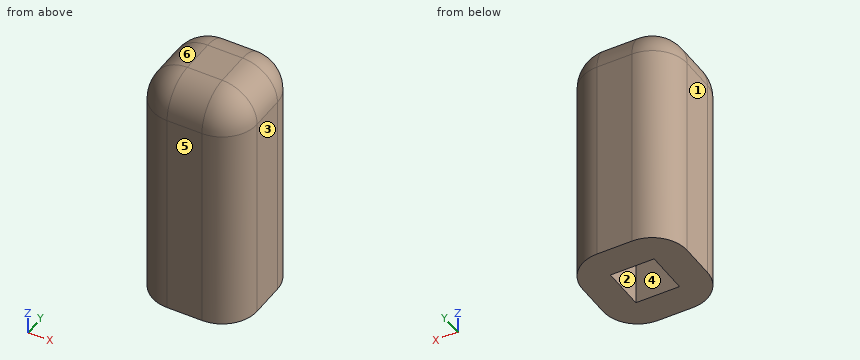
Autodesk Inventor part; units mm, degrees
ref_plane "YZ Plane" through (0, 0, 0) normal (1, 0, 0) x (0, 1, 0)
ref_plane "XZ Plane" through (0, 0, 0) normal (0, 1, 0) x (-1, 0, 0)
ref_plane "XY Plane" through (0, 0, 0) normal (0, 0, 1) x (1, 0, 0)
sketch "Sketch1" plane through (0, 0, 0) normal (0, 0, 1) x (1, 0, 0)
  line L0 (-1, 1) -> (1, 1)
  line L1 (1, 1) -> (1, -1)
  line L2 (1, -1) -> (-1, -1)
  line L3 (-1, -1) -> (-1, 1)
  line L4 (-1, 1) -> (1, -1) construction
  line L5 (1, 1) -> (-1, -1) construction
  line L6 (3, 3) -> (-3, 3)
  line L7 (-3, 3) -> (-3, -3)
  line L8 (-3, -3) -> (3, -3)
  line L9 (3, -3) -> (3, 3)
  point P0 (0, 0)
  dimension "d0" = 2
  dimension "d1" = 2
  dimension "d2" = 2
extrude "Extrusion1" add sketch "Sketch1" along normal blind 14
sketch "Sketch2" plane through (0, 0, 14) normal (0, 0, 1) x (1, 0, 0)
  line L0 (-3, -3) -> (3, -3)
  line L1 (3, -3) -> (3, 3)
  line L2 (3, 3) -> (-3, 3)
  line L3 (-3, 3) -> (-3, -3)
  line L4 (1, -1) -> (-1, -1)
  line L5 (-1, -1) -> (-1, 1)
  line L6 (-1, 1) -> (1, 1)
  line L7 (1, 1) -> (1, -1)
  point P0 (0, 0)
extrude "Extrusion2" add sketch "Sketch2" against normal blind 8 contours L4 L5 L6 L7
fillet "Fillet1" radius 2 8 edges at (3, 3, 7) (-3, 3, 7) (-3, -3, 7) (3, -3, 7) (3, 0, 14) (0, -3, 14) (-3, 0, 14) (0, 3, 14)
sketch "Sketch3" plane through (0, 0, 0) normal (0, 0, -1) x (-1, 0, 0)
  arc A0 (1, -3) -> (3, -1) centre (1, -1) ccw
  line L0 (3, 1) -> (3, -1)
  arc A1 (3, 1) -> (1, 3) centre (1, 1) ccw
  line L1 (-1, 3) -> (1, 3)
  arc A2 (-1, 3) -> (-3, 1) centre (-1, 1) ccw
  line L2 (-3, -1) -> (-3, 1)
  arc A3 (-3, -1) -> (-1, -3) centre (-1, -1) ccw
  line L3 (1, -3) -> (-1, -3)
  line L4 (-1, -1) -> (1, -1)
  line L5 (-1, 1) -> (-1, -1)
  line L6 (1, 1) -> (-1, 1)
  line L7 (1, -1) -> (1, 1)
  line L8 (-1.25, -1.25) -> (1.25, -1.25)
  line L9 (1.25, -1.25) -> (1.25, 1.25)
  line L10 (1.25, 1.25) -> (-1.25, 1.25)
  line L11 (-1.25, 1.25) -> (-1.25, -1.25)
  point P0 (0, 0)
  dimension "d8" = 0.25
extrude "Extrusion3" cut sketch "Sketch3" against normal blind 6 contours L5 L6 L7 L4 | L11 L10 L9 L8
properties part number "switch cover"
Build history of the part. All positions in model axes, mm. Face numbers are marked on the shaded views. A direction names the side the tool comes from. Round coordinates to 2 decimals unless told otherwise and drop trailing zeros. Write each loop counter-clockwise with the first axis right and the second up, starting at its lowest first coordinate (ties: lowest second). Pieces come first, ordered by that corner, then holes. Notation, with made-up numbers: (-30, 46.25) - (0, 46.25) arc R22 cw to (0, 75.25) - close; hole circle Ø11 at (83, 57.25). An arc over 180 degrees is marked (long way). Answer as CSV lines item,"result".
Q1. Drill centre lines: probe 1 along Y at (x, z) = (-0.25, 4.25); probe 2 along Z at (x, y) = (0.55, -0.1). Where is each one in solid material? Low to high. Write a range as [from, to].
Report:
probe 1,"y = [-3, -1.25], [1.25, 3]"
probe 2,"z = [6, 14]"
Q2. Cut at C-C (z = 10.5). Write the cut outline in (x, y), and give its area (3 significant figures).
Report:
outline,"(-3, -1) arc R2 ccw to (-1, -3) - (1, -3) arc R2 ccw to (3, -1) - (3, 1) arc R2 ccw to (1, 3) - (-1, 3) arc R2 ccw to (-3, 1) - close"
area,"32.6 mm^2"
Q3. Tool access for the marked faces 1 and 2: list every direction of +Z, -Z, +X, -X, +Y, -Y with a clear straight run to the whole face (end or side of a thin tool).
Report:
face 1,"+Z, -Z, -X, +Y, -Y"
face 2,"-Z"
Q4. Drop a flat-ended pin along its axis: pin 1 (1 mm diameter, centred on y = 1.5, z = 8.5, fed in from -X). Give the stop position or say it passes through.
Report:
pin 1,"stops at x = -3"
Q5. Cut at A-A (z = 5.75). Write the cut outline in (x, y), and give its area (3 significant figures).
Report:
outline,"(-3, -1) arc R2 ccw to (-1, -3) - (1, -3) arc R2 ccw to (3, -1) - (3, 1) arc R2 ccw to (1, 3) - (-1, 3) arc R2 ccw to (-3, 1) - close; hole (-1.25, -1.25) - (1.25, -1.25) - (1.25, 1.25) - (-1.25, 1.25) - close"
area,"26.3 mm^2"
Q6. Cut at B-B (y = -0.75). Write the cut outline in (x, z), and give its area (3 significant figures).
Report:
outline,"(-3, 0) - (-1.25, 0) - (-1.25, 6) - (1.25, 6) - (1.25, 0) - (3, 0) - (3, 12) arc R2 ccw to (1, 14) - (-1, 14) arc R2 ccw to (-3, 12) - close"
area,"67.3 mm^2"
Q7. Cut at D-D (x = 2.55). Write the cut outline in (y, z).
Report:
outline,"(-2.26, 0) - (2.26, 0) - (2.26, 12) arc R1.26 ccw to (1, 13.26) - (-1, 13.26) arc R1.26 ccw to (-2.26, 12) - close"
Q8. Pull direction X, two halves, no side cores. Call the marked faces 3, 4, 5 and 6: +X half, -X half, draft (parallel to the pull), parting line (faces both ways), or undercut.
Report:
face 3,"+X half"
face 4,"undercut"
face 5,"draft"
face 6,"-X half"
